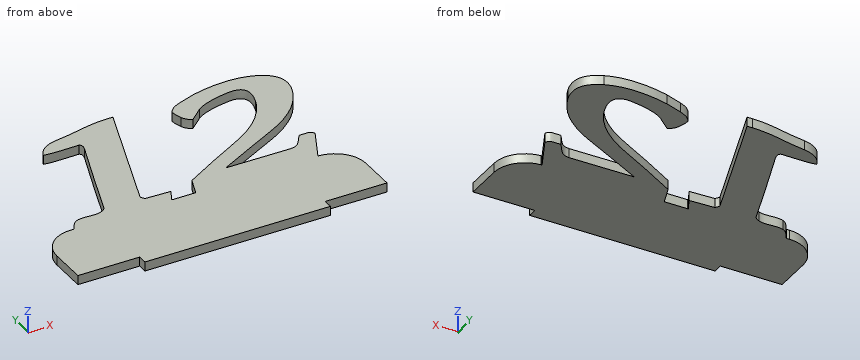
```python
from build123d import *

# Parameters (mm, degrees)
BOSS_EXTRUDE1_DEPTH = 3
FILLET1_R           = 10
FILLET2_R           = 0.2


with BuildPart() as part:
    # Sketch1 → Boss-Extrude1 (new body)
    with BuildSketch(Plane.XY):
        with BuildLine():
            Line((42.537984076, 22.000000982), (50.584636746, 22.000000982))
            Line((50.584636746, 22.000000982), (52.839649235, 28.197109379))
            add(Edge.make_bspline(
                [(52.839649235, 28.197109379), (54.248714684, 29.045506519), (56.431909075, 30.357383962), (59.474309712, 32.090120544), (61.944850647, 33.524828625), (64.570783761, 34.985747142), (67.336324518, 36.511397195), (70.231324588, 38.121508187), (73.255007633, 39.710376785), (76.200009812, 41.39768715), (78.906567156, 43.225136503), (81.348027085, 45.112569426), (83.490641674, 47.118195151), (85.357416855, 49.206298383), (87.428198995, 52.081305478), (88.630794744, 54.409507668), (89.196177773, 56.031354884)],
                knots=[0, 0, 0, 0, 0.105524725, 0.163385995, 0.224617296, 0.288806203, 0.356161699, 0.427252852, 0.501313646, 0.575301268, 0.644861957, 0.710669145, 0.773069231, 0.832880115, 0.890073183, 1, 1, 1, 1], degree=3))
            add(Edge.make_bspline(
                [(89.196177773, 56.031354884), (89.625842409, 57.266839405), (90.155099381, 59.015505319), (90.105779781, 61.237355295), (89.66646939, 62.439251642), (88.84893126, 63.338971158), (87.635580146, 63.810940124), (86.136489342, 63.992093331), (84.396326749, 63.803607869), (82.578344606, 63.493806461), (80.812926713, 63.154877277), (79.204447684, 62.73821432), (77.736657379, 62.289804925), (76.402583676, 61.814244169), (74.896898698, 61.102776297), (73.866127773, 60.496052109), (73.285309908, 59.99929859)],
                knots=[0, 0, 0, 0, 0.163533838, 0.22358703, 0.273097817, 0.319542769, 0.369979931, 0.431293779, 0.506061157, 0.586526579, 0.660902098, 0.729494961, 0.793064576, 0.851774175, 0.90542867, 1, 1, 1, 1], degree=3))
            Line((73.285309908, 59.99929859), (69.00462187, 56.226820091))
            add(Edge.make_bspline(
                [(69.00462187, 56.226820091), (68.473738468, 56.526672064), (67.547969563, 57.251968605), (66.901989109, 58.235224326), (66.698132425, 58.748321264)],
                knots=[0, 0, 0, 0, 0.525688222, 1, 1, 1, 1], degree=3))
            add(Edge.make_bspline(
                [(66.698132425, 58.748321264), (65.989020109, 60.529360233), (65.838085514, 62.44261368)],
                knots=[0, 0, 0, 1, 1, 1], degree=2))
            add(Edge.make_bspline(
                [(65.838085514, 62.44261368), (66.216607319, 63.204516033), (67.48287064, 64.66140426), (69.248688382, 65.425296692), (70.196959634, 65.804615243)],
                knots=[0, 0, 0, 0, 0.451020123, 1, 1, 1, 1], degree=3))
            add(Edge.make_bspline(
                [(70.196959634, 65.804615243), (72.817005486, 66.776950367), (75.474520228, 67.641988191)],
                knots=[0, 0, 0, 1, 1, 1], degree=2))
            add(Edge.make_bspline(
                [(75.474520228, 67.641988191), (77.097723123, 68.109547469), (79.616741412, 68.628507184), (83.063826554, 69.097528685), (85.75140454, 69.30616535), (88.452721605, 69.381691523), (91.938548042, 69.027238786), (94.465489273, 68.405808951), (96.057006546, 67.778813836)],
                knots=[0, 0, 0, 0, 0.242040332, 0.368376016, 0.498665213, 0.628561786, 0.755290793, 1, 1, 1, 1], degree=3))
            add(Edge.make_bspline(
                [(96.057006546, 67.778813836), (97.234318545, 67.300298489), (98.882536444, 66.423932293), (100.544073343, 64.729705469), (101.396826889, 63.351216745), (101.868398713, 61.797519742), (102.045609891, 59.41443702), (101.629471012, 57.577060636), (101.197741495, 56.363645736)],
                knots=[0, 0, 0, 0, 0.269969076, 0.3868787, 0.498157891, 0.609266408, 0.726758964, 1, 1, 1, 1], degree=3))
            add(Edge.make_bspline(
                [(101.197741495, 56.363645736), (100.627905221, 54.705185204), (99.401800162, 52.344246797), (97.33010629, 49.432482993), (95.47843029, 47.345736731), (93.329490859, 45.400929794), (90.938970266, 43.534651518), (88.270428499, 41.790403458), (84.397423166, 39.705285051), (79.587729815, 37.28204241), (72.604067537, 33.62463429), (67.574334477, 31.023637696), (64.39164298, 29.31126106)],
                knots=[0, 0, 0, 0, 0.112095574, 0.169586155, 0.228763596, 0.290550216, 0.355136688, 0.423026188, 0.494632822, 0.636984017, 0.768320184, 1, 1, 1, 1], degree=3))
            Line((64.39164298, 29.31126106), (85.423699274, 29.193981936))
            add(Edge.make_bspline(
                [(85.423699274, 29.193981936), (86.082600666, 29.252133566), (87.056534892, 29.476510222), (88.110965689, 30.221368973), (89.344492612, 31.708414679), (90.132287268, 33.128468355), (90.896725076, 34.19789124)],
                knots=[0, 0, 0, 0, 0.257232278, 0.374596102, 0.492310467, 1, 1, 1, 1], degree=3))
            add(Edge.make_bspline(
                [(90.896725076, 34.19789124), (91.748722118, 34.159580523), (92.786549209, 34.246487699), (94.041100815, 34.199570399), (94.810812918, 33.848834983), (95.196520755, 33.322492941), (95.392424841, 32.946913914)],
                knots=[0, 0, 0, 0, 0.506825366, 0.628241153, 0.743426283, 1, 1, 1, 1], degree=3))
            Line((95.392424841, 32.946913914), (90.110220598, 22.000000982))
            Line((90.110220598, 22.000000982), (100, 22.000000982))
            Line((100, 22.000000982), (100, 0))
            Line((100, 0), (80, 0))
            Line((80, 0), (80, -3))
            Line((80, -3), (20, -3))
            Line((20, -3), (20, 0))
            Line((20, 0), (0, 0))
            Line((0, 0), (0, 22.000000982))
            Line((0, 22.000000982), (11.126314779, 22.000000982))
            add(Edge.make_bspline(
                [(11.126314779, 22.000000982), (11.179175101, 22.091287797), (11.479303034, 22.615987108), (12.260783592, 24.017880313), (13.255402926, 25.187491124), (14.196177773, 25.616968644)],
                knots=[0.196060683, 0.196060683, 0.196060683, 0.196060683, 0.24891213, 0.498932816, 1, 1, 1, 1], degree=3))
            add(Edge.make_bspline(
                [(14.196177773, 25.616968644), (15.537546067, 26.136232655), (18.288283832, 25.861464595), (21.057617255, 25.705816495), (22.366623434, 26.281550349)],
                knots=[0, 0, 0, 0, 0.501451854, 1, 1, 1, 1], degree=3))
            add(Edge.make_bspline(
                [(22.366623434, 26.281550349), (23.248166371, 26.672062902), (23.949891612, 27.337062468)],
                knots=[0, 0, 0, 1, 1, 1], degree=2))
            add(Edge.make_bspline(
                [(23.949891612, 27.337062468), (25.732187491, 32.372235468), (29.257184693, 42.495036723), (32.946212686, 52.559233475), (34.778664091, 57.614623062)],
                knots=[0, 0, 0, 0, 0.498322561, 1, 1, 1, 1], degree=3))
            add(Edge.make_bspline(
                [(34.778664091, 57.614623062), (34.961841156, 58.112161275), (35.257027284, 59.078737049), (34.804433512, 59.990132521), (34.446373238, 60.194763797)],
                knots=[0, 0, 0, 0, 0.581397084, 1, 1, 1, 1], degree=3))
            add(Edge.make_bspline(
                [(34.446373238, 60.194763797), (32.529652356, 60.228560869), (28.724661476, 60.044652466), (24.911679757, 60.149389343), (23.031205138, 60.390229004)],
                knots=[0, 0, 0, 0, 0.503014916, 1, 1, 1, 1], degree=3))
            add(Edge.make_bspline(
                [(23.031205138, 60.390229004), (23.263167648, 61.057401499), (23.747411258, 62.006355534), (24.665405373, 63.067091706), (25.438689115, 63.789616743), (26.386650807, 64.343325333), (27.813668818, 65.026024955), (29.005726498, 65.340841829), (29.833394349, 65.472324391)],
                knots=[0, 0, 0, 0, 0.237267367, 0.352023708, 0.469658656, 0.590380818, 0.718477308, 1, 1, 1, 1], degree=3))
            add(Edge.make_bspline(
                [(29.833394349, 65.472324391), (32.945660374, 65.870761534), (36.807427968, 66.722765492), (41.429227523, 67.802579697), (44.509128617, 68.285055442), (46.80221991, 68.432605881), (48.304856428, 68.44339554)],
                knots=[0, 0, 0, 0, 0.501477793, 0.632810111, 0.759518477, 1, 1, 1, 1], degree=3))
            add(Edge.make_bspline(
                [(48.304856428, 68.44339554), (48.513352649, 68.44339554), (49.106263778, 68.44339554), (49.699174906, 68.44339554), (50.083589814, 68.44339554)],
                knots=[0, 0, 0, 0, 0.351648352, 1, 1, 1, 1], degree=3))
            Line((50.083589814, 68.44339554), (35.834176209, 27.806178965))
            add(Edge.make_bspline(
                [(35.834176209, 27.806178965), (35.780993555, 27.60638247), (36.11263329, 27.096689411), (36.390323638, 26.613906537), (36.694223121, 26.340189911)],
                knots=[0, 0, 0, 0, 0.324502414, 1, 1, 1, 1], degree=3))
            Line((36.694223121, 26.340189911), (44.864668782, 26.02744558))
            add(Edge.make_bspline(
                [(44.864668782, 26.02744558), (44.269729217, 25.014226453), (43.724569108, 23.691987076), (42.904365523, 22.352776547), (42.628440441, 22.079744483), (42.537984076, 22.000000982)],
                knots=[0, 0, 0, 0, 0.504343167, 0.619768133, 0.671675172, 0.671675172, 0.671675172, 0.671675172], degree=3))
        make_face()
    extrude(amount=BOSS_EXTRUDE1_DEPTH)

    # Fillet1
    # the kernel refuses this fillet: 10 mm, written as the material it takes off along each edge
    with BuildSketch(Plane(origin=(100, 22.000000982, -25), x_dir=(-1, 0, 0), z_dir=(0, 0, 1))) as fillet1_piece_1_section:
        with BuildLine():
            CenterArc((FILLET1_R, FILLET1_R), FILLET1_R, 180, 90)
            Line((0, FILLET1_R), (0, 0))
            Line((0, 0), (FILLET1_R, 0))
        make_face()
    fillet1_piece_1 = extrude(amount=53, mode=Mode.PRIVATE)
    fillet1_piece_1 = split(fillet1_piece_1, bisect_by=Plane(origin=(90.664979053, 23.149690057, 1.5), z_dir=(0.9006325457122767, -0.4345814280475224, 0)), keep=Keep.TOP, mode=Mode.PRIVATE)
    add(fillet1_piece_1, mode=Mode.SUBTRACT)
    with BuildSketch(Plane(origin=(0, 22.000000982, -25), x_dir=(0, -1, 0), z_dir=(0, 0, 1))) as fillet1_piece_2:
        with BuildLine():
            CenterArc((FILLET1_R, FILLET1_R), FILLET1_R, 180, 90)
            Line((0, FILLET1_R), (0, 0))
            Line((0, 0), (FILLET1_R, 0))
        make_face()
    extrude(amount=53, mode=Mode.SUBTRACT)

    # Fillet2
    fillet2_edges = [part.edges().sort_by_distance(p)[0] for p in [
        (90.109929036, 21.999396745, 1.5),
        (42.537984076, 22.000000982, 1.5),
        (50.584636746, 22.000000982, 1.5),
        (11.126314779, 22.000000982, 1.5),
    ]]
    fillet(fillet2_edges, radius=FILLET2_R)


solid = part.part
```
Could you check a few things on this model? Use its own coordinates, in mm. Give positions to 0.01 mm unless a question says otherwise; leave off trailing zeros. Write each loop counter-clockwise with the first axis right and the second up, starting at its lowest first coordinate (ties: lowest second). Pieces come first, ordered by that corner, then holes. Notation, with made-up numbers: (60.25, -22) - (67.25, -22) arc R13 cw to (67.25, -10) - close; hole circle Ø10 at (10.25, 53). An arc over 180 degrees is marked (long way). One line per item, written item: value. Start each with the question number.
Item 1: Imagine slicing it at A-A, the plane y = 10.5. List the corners of the cut face in (x, z) for me.
Item 2: I'm going to push flat-ended pins straight in: pin 1 (1.5 mm diameter, centred on y = 54.5, z = 1.5, fed in from +X); pin 2 (0.8 mm diameter, centred on x = 10.5, z = 2, fed in from +Y); pin 3 (1.5 mm diameter, centred on x = 95, z = 1, fed in from -Y). Where does each tip first touch, or does it pass through?
Item 3: Please list where these lines run through material, in increasing order: line 1 (X direction, y = 30, z = 2.45); line 2 (X direction, y = 59.5, z = 1.7); line 3 (Y direction, x = 67.5, z = 2.2). Write a range as from..to.
Item 4: Imagine slicing it at B-B, the plane y = 31. Give the number of separate pieces and of enclosed holes in the cut face, and give its area (3 significant figures).
Geometry says:
1. outline: (0, 0) - (100, 0) - (100, 3) - (0, 3) - close
2. pin 1: x = 100.77
2. pin 2: y = 22
2. pin 3: y = 0
3. line 1: 24.89..36.6, 55.85..65.68, 87.78..93.97
3. line 2: 34.99..46.95, 66.43..72.72, 90.07..101.91
3. line 3: -3..29.29, 30.97..36.6, 57.45..64.41
4. separate pieces: 3
4. enclosed holes: 0
4. area: 82.3 mm^2
